For this review, take the finished solid that the model builds, in its own axes (mm). Give positions to 0.01 mm unless a question says otherwise; leave off trailing zeros. Loops run counter-clockwise (first coordinate to the right, second up) from the corner with the lowest first, then second, coordinate; pieces in that order, holes last. Notation, with made-up numbers: (46.5, -2.75) - (53.5, -2.75) arc R16 cw to (53.5, 27.25) - close; hole circle Ø1 at (-1.5, 76.25). An arc over 180 degrees is marked (long way). Answer in a Markdown table with one row per item.
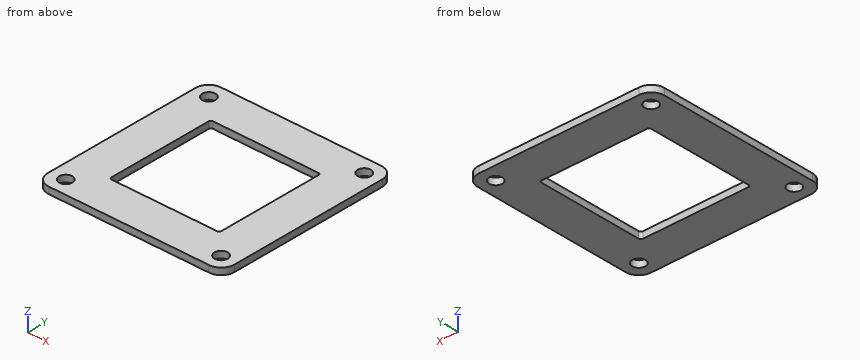
Autodesk Inventor part; units mm, degrees
ref_plane "YZ Plane" through (0, 0, 0) normal (1, 0, 0) x (0, 1, 0)
ref_plane "XZ Plane" through (0, 0, 0) normal (0, 1, 0) x (-1, 0, 0)
ref_plane "XY Plane" through (0, 0, 0) normal (0, 0, 1) x (1, 0, 0)
sketch "Sketch1" plane through (0, 0, 0) normal (0, 0, 1) x (1, 0, 0)
  line L0 (-42.5, -42.5) -> (42.5, -42.5)
  line L1 (42.5, -42.5) -> (42.5, 42.5)
  line L2 (42.5, 42.5) -> (-42.5, 42.5)
  line L3 (-42.5, 42.5) -> (-42.5, -42.5)
  line L4 (-42.5, -42.5) -> (42.5, 42.5) construction
  line L5 (42.5, -42.5) -> (-42.5, 42.5) construction
  line L6 (25, -25) -> (-25, -25)
  line L7 (-25, -25) -> (-25, 25)
  line L8 (-25, 25) -> (25, 25)
  line L9 (25, 25) -> (25, -25)
  line L10 (25, -25) -> (-25, 25) construction
  line L11 (-25, -25) -> (25, 25) construction
  point P0 (0, 0)
  dimension "d154" = 85
  dimension "d155" = 85
  dimension "d172" = 50
extrude "Plate5" add sketch "Sketch1" along normal blind 3
sketch "Sketch9" plane through (0, 0, 3) normal (0, 0, 1) x (1, 0, 0)
  circle A0 centre (35.3553, -35.3553) radius 3
  line L0 (35.3553, 35.3553) -> (-35.3553, 35.3553) construction
  line L1 (-35.3553, 35.3553) -> (-35.3553, -35.3553) construction
  line L2 (-35.3553, -35.3553) -> (35.3553, -35.3553) construction
  line L3 (35.3553, -35.3553) -> (35.3553, 35.3553) construction
  line L4 (35.3553, 35.3553) -> (-35.3553, -35.3553) construction
  line L5 (-35.3553, 35.3553) -> (35.3553, -35.3553) construction
  circle A1 centre (-35.3553, -35.3553) radius 3
  circle A2 centre (35.3553, 35.3553) radius 3
  circle A3 centre (-35.3553, 35.3553) radius 3
  circle A4 centre (0, 0) radius 50 construction
  dimension "d180" = 100
  dimension "d174" = 6
extrude "Cut2" cut sketch "Sketch9" against normal blind 3
fillet "Corner Round1" radius 6 4 edges at (42.5, 42.5, 1.5) (-42.5, 42.5, 1.5) (-42.5, -42.5, 1.5) (42.5, -42.5, 1.5)
fillet "Corner Round2" radius 1 4 edges at (-25, 25, 1.5) (-25, -25, 1.5) (25, -25, 1.5) (25, 25, 1.5)
properties part number "TKS 3531 FDS Way FLANGE" material "Stainless Steel"
1. Wall thickness on line 1 (Y direction, x = -35.5, z = 2.1); line 2 (Y direction, x = 23, z = 1.7): over which ranges is each line inside the solid? List them lowest first. Write a range as [from, to].
Values:
| item | result |
|---|---|
| line 1 | y = [-42.5, -38.35], [-32.36, 32.36], [38.35, 42.5] |
| line 2 | y = [-42.5, -25], [25, 42.5] |
2. We need section A-A, the plane x = -6.5. Give the boundary of the cut face in (y, z), and give its area (3 significant figures).
Values:
| item | result |
|---|---|
| outline | (-42.5, 0) - (-25, 0) - (-25, 3) - (-42.5, 3) - close; (25, 0) - (42.5, 0) - (42.5, 3) - (25, 3) - close |
| area | 105 mm^2 |
3. We need section C-C, the plane z = 2.35. Give the boundary of the cut face in (x, y).
Values:
| item | result |
|---|---|
| outline | (-42.5, -36.5) arc R6 ccw to (-36.5, -42.5) - (36.5, -42.5) arc R6 ccw to (42.5, -36.5) - (42.5, 36.5) arc R6 ccw to (36.5, 42.5) - (-36.5, 42.5) arc R6 ccw to (-42.5, 36.5) - close; hole circle Ø6 at (-35.36, -35.36); hole circle Ø6 at (-35.36, 35.36); hole (-25, -24) arc R1 ccw to (-24, -25) - (24, -25) arc R1 ccw to (25, -24) - (25, 24) arc R1 ccw to (24, 25) - (-24, 25) arc R1 ccw to (-25, 24) - close; hole circle Ø6 at (35.36, -35.36); hole circle Ø6 at (35.36, 35.36) |
4. Clearance check with a flat-ended pin moving along its axis: pin 1 (5 mm diameter, centred on x = 35.36, y = 35.36, fed in from -Z). State where the tip first meets the part, or that it passes through.
Values:
| item | result |
|---|---|
| pin 1 | passes through |
